The model under review builds one solid part; all positions refer to its coordinate system, in mm. Face numbers are marked on the shaded views. Round coordinates to 2 decimals unless told otherwise and drop trailing zeros. Write each loop counter-clockwise with the first axis right and the second up, starting at its lowest first coordinate (ties: lowest second). Pieces come first, ordered by that corner, then holes. Notation, with made-up numbers: (25.25, -26.5) -> (72.25, -26.5) arc R25 ccw to (72.25, -10.5) -> close; hole circle Ø2 at (41, 65). An arc over 180 degrees is marked (long way). Answer in a Markdown table with one row per item. Add a question column.
```python
from build123d import *

# Parameters (mm, degrees)
CUT_EXTRUDE7_REACH      = 103
SKETCH5_R               = 54
CUT_EXTRUDE8_REACH      = 103
SKETCH6_R               = 65
BOSS_EXTRUDE1_DEPTH     = 2
SKETCH9_R               = 6
CUT_EXTRUDE9_DEPTH      = 200
CUT_EXTRUDE9_DEPTH_BACK = 200
SKETCH10_R              = 7
CUT_EXTRUDE10_DEPTH     = 20


with BuildPart() as part:
    # Sketch2 → Globe (revolve)
    with BuildSketch(Plane(origin=(0, 0, 0), x_dir=(1, 0, 0), z_dir=(0, 1, 0))):
        with BuildLine():
            ThreePointArc((0, -101), (101, 0), (0, 101))
            Line((0, 101), (0, 99))
            ThreePointArc((0, 99), (99, 0), (0, -99))
            Line((0, -99), (0, -101))
        make_face()
    revolve(axis=Axis((0, 0, 100), (0, 0, -1)))

    # Sketch5 → Cut-Extrude7 (cut, up to next)
    with BuildSketch(Plane(origin=(0, 0, 0), x_dir=(1, 0, 0), z_dir=(0, 1, 0)), mode=Mode.PRIVATE) as cut_extrude7_sk1:
        Circle(SKETCH5_R)
    cut_extrude7_tool1 = extrude(cut_extrude7_sk1.sketch, amount=CUT_EXTRUDE7_REACH, mode=Mode.PRIVATE) & part.part
    add(cut_extrude7_tool1.solids().sort_by_distance((0, 0, 0))[0], mode=Mode.SUBTRACT)

    # Sketch6 → Cut-Extrude8 (cut, up to next)
    with BuildSketch(Plane.XY, mode=Mode.PRIVATE) as cut_extrude8_sk1:
        Circle(SKETCH6_R)
    cut_extrude8_tool1 = extrude(cut_extrude8_sk1.sketch, amount=CUT_EXTRUDE8_REACH, mode=Mode.PRIVATE) & part.part
    add(cut_extrude8_tool1.solids().sort_by_distance((0, 0, 0))[0], mode=Mode.SUBTRACT)

    # Sketch7 → Boss-Extrude1 (add)
    with BuildSketch(Plane(origin=(0, 85.352211453, 0), x_dir=(-1, 0, 0), z_dir=(0, -1, 0))):
        with BuildLine():
            Line((10, -53.065996646), (10, 53.065996646))
            ThreePointArc((10, 53.065996646), (-54, 0), (10, -53.065996646))
        make_face()
    extrude(amount=BOSS_EXTRUDE1_DEPTH)

    # Sketch9 → Cut-Extrude9 (cut, two sides)
    with BuildSketch(Plane(origin=(0, 0, 0), x_dir=(0, 0, -1), z_dir=(1, 0, 0))) as cut_extrude9_sk:
        Circle(SKETCH9_R)
    extrude(amount=CUT_EXTRUDE9_DEPTH, mode=Mode.SUBTRACT)
    extrude(cut_extrude9_sk.sketch, amount=-CUT_EXTRUDE9_DEPTH_BACK, mode=Mode.SUBTRACT)

    # Sketch10 → Cut-Extrude10 (cut)
    with BuildSketch(Plane(origin=(0, 85.352211453, 0), x_dir=(1, 0, 0), z_dir=(0, 1, 0))):
        with Locations((0, 27)):
            Circle(SKETCH10_R)
        with Locations((0, -27)):
            Circle(SKETCH10_R)
    extrude(amount=-CUT_EXTRUDE10_DEPTH, mode=Mode.SUBTRACT)


solid = part.part
```
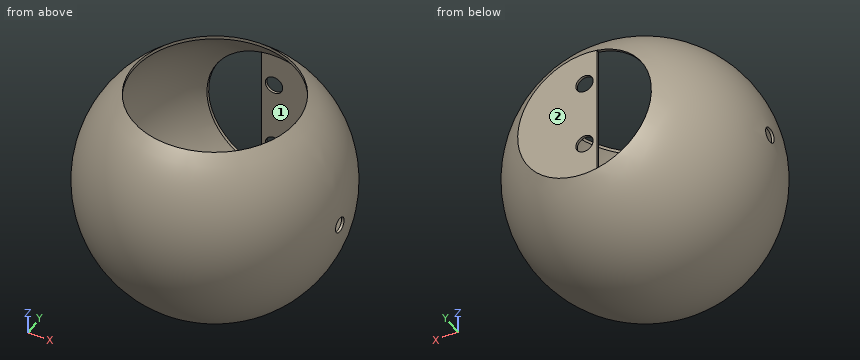
1. Mouldability with a two-part tool opening along Z and no side actions: class the marked faces 1 and 2 as pulls with the +Z half, pulls with the -Z half, needs draft (parallel to the pull), parting line crosses it, or undercut.
2. For L1, parallel to Z at x = 0, y = 84; L2, parallel to Y at x = 36.5, z = -83; L3, parallel to X at y = 71, z = 28, list the stretches that pass through material, from the lowest coordinate up.
3. Add section C-C on z = -27. Write out the cut boundary in (x, y).
4. Add section B-B on x = 0. Write out the cut boundary in (y, z), plus the area to 3 significant figures.
5. Insertion check: pin 1 Ø12 at (x, z) = (53.5, -40.5) entering from -Y; pin 2 Ø1 at (y, z) = (-49.5, -47.5) entering from +X; pin 3 Ø5 at (x, y) = (-77.5, -24.5) entering from +Z. Each pin has a flat end and moves straight along its axis. Give the tip position at first contact, or say it passes through.
Filled in:
| question | item | result |
|---|---|---|
| 1 | face 1 | undercut |
| 1 | face 2 | needs draft |
| 2 | L1 | -56.08 to -34, -20 to 20, 34 to 56.08 |
| 2 | L2 | -44.49 to -39.75, 39.75 to 44.49 |
| 2 | L3 | -66.15 to -63.06, 63.06 to 66.15 |
| 3 | outline | (-46.77, 82.98) -> (-46.77, 85.35) arc R97.32 ccw (long way) to (46.77, 85.35) -> (7, 85.35) -> (7, 83.35) -> (46.77, 83.35) -> (46.77, 82.98) arc R95.25 cw (long way) to start; (-10, 83.35) -> (-7, 83.35) -> (-7, 85.35) -> (-10, 85.35) -> close |
| 4 | outline | (-65, 74.67) -> (-65, 77.3) arc R101 ccw (long way) to (85.35, -54) -> (85.35, -34) -> (83.35, -34) -> (83.35, -54) -> (82.98, -54) arc R99 cw (long way) to start; (65, 74.67) arc R99 cw to (82.98, 54) -> (83.35, 54) -> (83.35, 34) -> (85.35, 34) -> (85.35, 54) arc R101 ccw to (65, 77.3) -> close; (83.35, -20) -> (85.35, -20) -> (85.35, 20) -> (83.35, 20) -> close |
| 4 | area | 905 mm² |
| 5 | pin 1 | y = -80.42 |
| 5 | pin 2 | x = 74.58 |
| 5 | pin 3 | z = 63.2 |
